The figure shows three views and two pictorial views of one solid part (mm, origin at its lowest corner). Answer the questions. A direction names the side the tool comes from. Coordinates: 2 decimals unless noted, no trailing zeros. Loops run counter-clockwise (first coordinate to the right, second up) from the corner with the lowest first, then second, coordinate; pieces in that order, holes last. Notation, with made-up numbers: M 0.5,27 L 20.5,27 A29 cw 20.5,57 Z; hole C 78.25,28.25 d9. An arc over 180 degrees is marked long. Write each question's results on one line, items separated by ' | '.
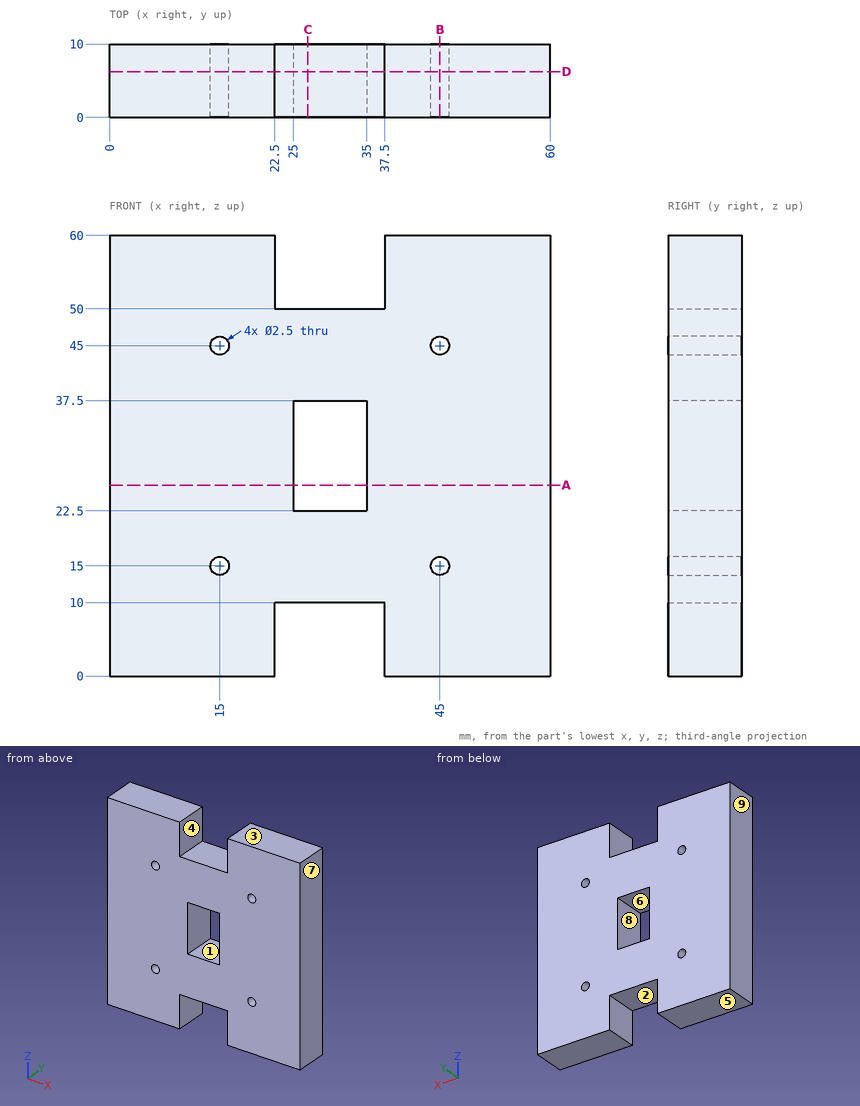
1) For a pull along X with two mould halves and no side action, classify the marked faces 6, 7, 8 and 9 as released by +X, released by -X, zero draft, split by the parting line, or undercut.
Check result:
face 6: undercut | face 7: released by +X | face 8: undercut | face 9: released by -X
2) Straight lines are drawn through the part: probe 1 along X at (y, z) = (6.75, 45); probe 2 along X at (y, z) = (1.5, 57.5); probe 3 along X at (y, z) = (6, 27). For each, find the intervals that lie inside material, in ascending order. Write a range as [from, to].
Check result:
probe 1: [0, 13.75], [16.25, 43.75], [46.25, 60] | probe 2: [0, 22.5], [37.5, 60] | probe 3: [0, 25], [35, 60]
3) Find section C-C, the plane x = 27. Give the vertices of the cut face in (y, z), and give its area (3 significant figures).
Check result:
outline: M 0,10 L 10,10 L 10,22.5 L 0,22.5 Z; M 0,37.5 L 10,37.5 L 10,50 L 0,50 Z | area: 250 mm^2
4) Find section A-A, the plane z = 26. Give the vertices of the cut face in (x, y), and give its area (3 significant figures).
Check result:
outline: M 0,0 L 25,0 L 25,10 L 0,10 Z; M 35,0 L 60,0 L 60,10 L 35,10 Z | area: 500 mm^2
5) Given pin 1 Ø3 at (x, z) = (15, 15) entering from -Y; pin 2 Ø5 at (x, y) = (32, 5.5) entering from +Z; pin 3 Ø1.5 at (x, z) = (15, 45) entering from -Y; pin 4 Ø3 at (x, y) = (27, 6) entering from -Z, each flat-ended and moving along its own axis, determine where each tip first touches the part or whether it passes through.
Check result:
pin 1: y = 0 | pin 2: z = 50 | pin 3: through | pin 4: z = 10
6) Find section B-B, the plane x = 45. Give the vertices of the cut face in (y, z), and give its area (3 significant figures).
Check result:
outline: M 0,0 L 10,0 L 10,13.75 L 0,13.75 Z; M 0,16.25 L 10,16.25 L 10,43.75 L 0,43.75 Z; M 0,46.25 L 10,46.25 L 10,60 L 0,60 Z | area: 550 mm^2
7) Which of the six approach directions +Z, -Z, +X, -X, +Y, -Y give full straight-line access (tool end or side, diameter ignored) to the marked faces 1, 2, 3, 4 and 5?
Check result:
face 1: +Y, -Y | face 2: -Z, +Y, -Y | face 3: +Z, +X, -X, +Y, -Y | face 4: +Z, +Y, -Y | face 5: -Z, +X, -X, +Y, -Y
8) Find section D-D, the plane y = 6.25. Give the vertices of the cut face in (x, z), and give its area (3 significant figures).
Check result:
outline: M 0,0 L 22.5,0 L 22.5,10 L 37.5,10 L 37.5,0 L 60,0 L 60,60 L 37.5,60 L 37.5,50 L 22.5,50 L 22.5,60 L 0,60 Z; hole C 15,15 d2.5; hole C 15,45 d2.5; hole M 25,22.5 L 35,22.5 L 35,37.5 L 25,37.5 Z; hole C 45,15 d2.5; hole C 45,45 d2.5 | area: 3,130 mm^2
